from build123d import *

# Parameters (mm, degrees)
EXTRUDE_1_DEPTH     = 20
SKETCH_2_W          = 100
SKETCH_2_H          = 40
CUT_EXTRUDE_1_DEPTH = 20
FILLET_1_R          = 15
SKETCH_3_W          = 110
SKETCH_3_H          = 160
CUT_EXTRUDE_2_DEPTH = 10


with BuildPart() as part:
    # 스케치1 → 보스-돌출1 (new body)
    with BuildSketch(Plane(origin=(0, 0, 0), x_dir=(1, 0, 0), z_dir=(0, 1, 0))):
        Polygon((-65, 90), (-65, -90), (65, -90), (65, 90), (30, 90), (30, 110), (-30, 110), (-30, 90), align=None)
    extrude(amount=EXTRUDE_1_DEPTH)

    # 스케치2 → 컷-돌출1 (cut)
    with BuildSketch(Plane(origin=(0, 20, 0), x_dir=(1, 0, 0), z_dir=(0, 1, 0))):
        with Locations((0, -55)):
            Rectangle(SKETCH_2_W, SKETCH_2_H)
        with Locations((0, 55)):
            Rectangle(SKETCH_2_W, SKETCH_2_H)
        Rectangle(SKETCH_2_W, SKETCH_2_H)
    extrude(amount=-CUT_EXTRUDE_1_DEPTH, mode=Mode.SUBTRACT)

    # 필렛1
    fillet_1_edges = [part.edges().sort_by_distance(p)[0] for p in [
        (65, 10, -90),
        (65, 10, 90),
        (-65, 10, 90),
        (-65, 10, -90),
    ]]
    fillet(fillet_1_edges, radius=FILLET_1_R)

    # 스케치3 → 컷-돌출2 (cut)
    with BuildSketch(Plane.XZ):
        Rectangle(SKETCH_3_W, SKETCH_3_H)
    extrude(amount=-CUT_EXTRUDE_2_DEPTH, mode=Mode.SUBTRACT)


solid = part.part
Work out the finished part from the listing and answer in its coordinate system (mm). A direction names the side the tool comes from. Round coordinates to 2 decimals unless told otherwise and drop trailing zeros. Order: outer loops, then holes, each group sorted by start corner. A loop starts at its lowest first (then second) coordinate and runs counter-clockwise, first axis right, second up. Notation, with made-up numbers: M 32.5,67 L 69.5,67 A28 cw 69.5,104 Z; hole C 58.5,-35.5 d7. An arc over 180 degrees is marked long. Put each result on its own line as item: value. Start each with the question number.
Q1. A tool of negligible diameter and unlimited length cuts with its end or side. For faces 1 (the flat face through (40, 10, -90)), 2 (the flat face through (-1, 5, 80)), 3 (the flat face through (-1, 20, -34)), 4 (the flat face through (-40, 10, -90)), 5 (the flat face through (-1, 15, 35)), from which of +Z, -Z, +X, -X, +Y, -Y can it reach the whole face along a straight path? Write none if from no direction.
Q2. Section C-C, the plane y = 17.75 is taken. Write down the section's boundary in (x, z), and give its area (3 significant figures).
Q3. Section A-A, the plane x = -42.5 is taken. Write down the section's boundary in (y, z).
Q4. For a pull along X with two mould halves and no side action, classify faces 6 (the flat face through (-1, 5, -80)), 7 (the flat face through (-1, 15, 75)), 8 (the cylindrical face through (-60.72, 10.14, 85.49)), 9 (the cylindrical face through (60.49, 10.14, 85.72)) as pulls with the +X half, pulls with the -X half, needs draft (parallel to the pull), parting line crosses it, or undercut.
Q5. Section D-D, the plane y = 4.75 is taken. Write down the section's boundary in (x, z), and give its area (3 significant figures).
Q6. Straight lines are drawn through the part: L1, parallel to Z at x = 31, y = 13.5; L2, parallel to Z at x = -28.5, y = 17.5; L3, parallel to X at y = 14, z = 38. For each, find the intervals that lie inside material, in ascending order. Write a range as [from, to].
Q7. Section B-B, the plane z = -68 is taken. Write down the section's boundary in (x, y), and give its area (3 significant figures).
Q8. Flat-ended cylindrical pins translate along their axes: pin 1 (4 mm diameter, centred on x = 48, y = 6.5, fed in from -Z); pin 2 (1.5 mm diameter, centred on x = 38.5, z = 26.5, fed in from -Y); pin 3 (10 mm diameter, centred on y = 12.5, z = -102.5, fed in from -X). Find the tip coordinate at first contact, or state that the pin passes through.
Findings below:
1. face 1: -Z, +X, +Y, -Y
1. face 2: -Y
1. face 3: +Z, -Z, +X, -X, +Y
1. face 4: -Z, -X, +Y, -Y
1. face 5: +Y, -Y
2. outline: M -65,-75 A15 ccw -50,-90 L -30,-90 L -30,-110 L 30,-110 L 30,-90 L 50,-90 A15 ccw 65,-75 L 65,75 A15 ccw 50,90 L -50,90 A15 ccw -65,75 Z; hole M -50,-75 L 50,-75 L 50,-35 L -50,-35 Z; hole M -50,-20 L 50,-20 L 50,20 L -50,20 Z; hole M -50,35 L 50,35 L 50,75 L -50,75 Z
2. area: 12,400 mm^2
3. outline: M 0,-90 L 20,-90 L 20,-75 L 10,-75 L 10,-80 L 0,-80 Z; M 0,80 L 10,80 L 10,75 L 20,75 L 20,90 L 0,90 Z; M 10,-35 L 20,-35 L 20,-20 L 10,-20 Z; M 10,20 L 20,20 L 20,35 L 10,35 Z
4. face 6: undercut
4. face 7: undercut
4. face 8: pulls with the -X half
4. face 9: pulls with the +X half
5. outline: M -65,-75 A15 ccw -50,-90 L -30,-90 L -30,-110 L 30,-110 L 30,-90 L 50,-90 A15 ccw 65,-75 L 65,75 A15 ccw 50,90 L -50,90 A15 ccw -65,75 Z; hole M -55,-80 L 55,-80 L 55,80 L -55,80 Z
5. area: 6,810 mm^2
6. L1: z = [-90, -75], [-35, -20], [20, 35], [75, 90]
6. L2: z = [-110, -75], [-35, -20], [20, 35], [75, 90]
6. L3: x = [-65, -50], [50, 65]
7. outline: M -65,0 L -55,0 L -55,10 L -50,10 L -50,20 L -65,20 Z; M 50,10 L 55,10 L 55,0 L 65,0 L 65,20 L 50,20 Z
7. area: 500 mm^2
8. pin 1: stops at z = -90
8. pin 2: stops at y = 10
8. pin 3: stops at x = -30
